CAD build for the part. Positions are in the model's coordinates, mm. A direction names the side the tool comes from. Round coordinates to 2 decimals unless told otherwise and drop trailing zeros. Order: outer loops, then holes, each group sorted by start corner. A loop starts at its lowest first (then second) coordinate and runs counter-clockwise, first axis right, second up.
```python
from build123d import *

# Parameters (mm, degrees)
SKETCH1_W           = 9.5
SKETCH1_H           = 16.65
BOSS_EXTRUDE1_DEPTH = 0.2
SKETCH1_3_W         = 0.5
SKETCH1_3_H         = 0.5
BOSS_EXTRUDE2_DEPTH = 2
SKETCH1_4_W         = 9.5
SKETCH1_4_H         = 14.9
SKETCH1_4_W_2       = 9.1
SKETCH1_4_H_2       = 14.5
BOSS_EXTRUDE3_DEPTH = 0.25
BOSS_EXTRUDE4_DEPTH = 2
SKETCH1_6_W         = 0.670753581
SKETCH1_6_H         = 1.75
SKETCH1_6_W_2       = 1.029246419
SKETCH1_6_H_2       = 0.5
SKETCH1_6_W_3       = 3.329246419
BOSS_EXTRUDE5_DEPTH = 2
FILLET1_R           = 0.1
BOSS_EXTRUDE6_DEPTH = 0.2
SKETCH1_10_W        = 3.329246419
SKETCH1_10_H        = 0.5
SKETCH1_10_W_2      = 0.670753581
SKETCH1_10_H_2      = 1.75
BOSS_EXTRUDE7_DEPTH = 2
CUT_EXTRUDE1_DEPTH  = 18.429429136


with BuildPart() as part:
    # Sketch1 → Boss-Extrude1 (new body)
    with BuildSketch(Plane(origin=(0, 0, 0), x_dir=(1, 0, 0), z_dir=(0, 1, 0))):
        with Locations((0, -0.875)):
            Rectangle(SKETCH1_W, SKETCH1_H)
        Polygon((-3.55, 6.25), (3.05, 6.25), (3.05, 5.75), (3.55, 5.75), (3.55, -5.75), (3.05, -5.75), (3.05, -6.25), (-3.05, -6.25), (-3.05, -5.75), (-3.55, -5.75), align=None, mode=Mode.SUBTRACT)
    extrude(amount=-BOSS_EXTRUDE1_DEPTH)

    # Sketch1_3 → Boss-Extrude2 (add)
    with BuildSketch(Plane(origin=(0, 0, 0), x_dir=(1, 0, 0), z_dir=(0, 1, 0))):
        with Locations((3.3, -6)):
            Rectangle(SKETCH1_3_W, SKETCH1_3_H)
        with Locations((3.3, 6)):
            Rectangle(SKETCH1_3_W, SKETCH1_3_H)
        with Locations((-3.3, -6)):
            Rectangle(SKETCH1_3_W, SKETCH1_3_H)
    extrude(amount=-BOSS_EXTRUDE2_DEPTH)

    # Sketch1_4 → Boss-Extrude3 (add)
    with BuildSketch(Plane(origin=(0, 0, 0), x_dir=(1, 0, 0), z_dir=(0, 1, 0))):
        Rectangle(SKETCH1_4_W, SKETCH1_4_H)
        Rectangle(SKETCH1_4_W_2, SKETCH1_4_H_2, mode=Mode.SUBTRACT)
    extrude(amount=BOSS_EXTRUDE3_DEPTH)

    # Sketch1_5 → Boss-Extrude4 (add)
    with BuildSketch(Plane(origin=(0, 0, 0), x_dir=(1, 0, 0), z_dir=(0, 1, 0))):
        Polygon((-4.75, 7.45), (-4.75, -7.45), (-3.05, -7.45), (-3.05, -6.25), (-3.55, -6.25), (-3.55, 6.25), (-3.05, 6.25), (-3.05, 7.45), align=None)
        Polygon((3.55, -6.25), (3.05, -6.25), (3.05, -6.95), (4.079246419, -6.95), (4.079246419, -7.45), (4.75, -7.45), (4.75, 7.45), (4.079246419, 7.45), (4.079246419, 6.95), (3.05, 6.95), (3.05, 6.25), (3.55, 6.25), align=None)
    extrude(amount=-BOSS_EXTRUDE4_DEPTH)

    # Sketch1_6 → Boss-Extrude5 (add)
    with BuildSketch(Plane(origin=(0, 0, 0), x_dir=(1, 0, 0), z_dir=(0, 1, 0))):
        with Locations((-4.41462321, -8.325)):
            Rectangle(SKETCH1_6_W, SKETCH1_6_H)
        with Locations((3.56462321, 7.2)):
            Rectangle(SKETCH1_6_W_2, SKETCH1_6_H_2)
        with Locations((2.41462321, -7.2)):
            Rectangle(SKETCH1_6_W_3, SKETCH1_6_H_2)
        with Locations((4.41462321, -8.325)):
            Rectangle(SKETCH1_6_W, SKETCH1_6_H)
    extrude(amount=-BOSS_EXTRUDE5_DEPTH)

    # Fillet1
    fillet1_edges = [part.edges().sort_by_distance(p)[0] for p in [
        (3.05, -1.1, 6.95),
    ]]
    fillet(fillet1_edges, radius=FILLET1_R)

    # Sketch1_9 → Boss-Extrude6 (add)
    with BuildSketch(Plane(origin=(0, 0, 0), x_dir=(1, 0, 0), z_dir=(0, 1, 0))):
        Polygon((-4.079246419, 9.2), (-4.079246419, 7.45), (-3.05, 7.45), (0, 7.45), (0.75, 7.45), (3.05, 7.45), (4.079246419, 7.45), (4.079246419, 8.7), (0.75, 8.7), (0.75, 9.2), align=None)
    extrude(amount=-BOSS_EXTRUDE6_DEPTH)

    # Sketch1_10 → Boss-Extrude7 (add)
    with BuildSketch(Plane(origin=(0, 0, 0), x_dir=(1, 0, 0), z_dir=(0, 1, 0))):
        with Locations((2.41462321, 8.95)):
            Rectangle(SKETCH1_10_W, SKETCH1_10_H)
        Polygon((4.75, 9.2), (4.079246419, 9.2), (4.079246419, 8.7), (4.079246419, 7.45), (4.75, 7.45), align=None)
        with Locations((-4.41462321, 8.325)):
            Rectangle(SKETCH1_10_W_2, SKETCH1_10_H_2)
    extrude(amount=-BOSS_EXTRUDE7_DEPTH)

    # Sketch6 → Cut-Extrude1 (cut, through all)
    with BuildSketch(Plane.XY.offset(7.45)):
        with BuildLine():
            Line((-4.079246419, -2), (-3.779246419, -2))
            Line((-3.779246419, -2), (-3.779246419, -1.8))
            ThreePointArc((-3.779246419, -1.8), (-3.808535741, -1.729289322), (-3.879246419, -1.7))
            Line((-3.879246419, -1.7), (-3.979246419, -1.7))
            ThreePointArc((-3.979246419, -1.7), (-4.049957097, -1.729289322), (-4.079246419, -1.8))
            Line((-4.079246419, -1.8), (-4.079246419, -2))
        make_face()
    cut_extrude1 = extrude(amount=-CUT_EXTRUDE1_DEPTH, mode=Mode.SUBTRACT)

    # Mirror1: Cut-Extrude1 across plane
    add(cut_extrude1.mirror(Plane(origin=(0, 0, 0), x_dir=(0, 0, 1), z_dir=(1, 0, 0))), mode=Mode.SUBTRACT)


solid = part.part
```
1. Cut at D-D, the plane x = -2.5. Write the cut outline in (y, z).
2. Drill centre lines: line 1 (X direction, y = -0.2, z = 6); line 2 (Z direction, x = 2.5, y = -1.5); line 3 (X direction, y = -1.75, z = 0.5). Where is each one in solid material? Low to high.
3. Mould opens along X. For faces 1 (the face through (-4, 0, 0)), 2 (the face through (0, 0, 8)), 3 (the face through (2, -1, -8.7)), 4 (the face through (4.75, -1, 0)) say: released by +X, released by -X, zero draft, split by the parting line, or undercut.
4. Cut at C-C, the plane x = 1.25. Write the cut outline in (y, z), and give its area (3 significant figures).
5. Cut at A-A, the plane z = -1.5. Write the cut outline in (x, y), and give its area (3 significant figures).
6. Pin check, flat tips, straight feed: P1, Ø0.8, axis at x = -3.5, y = -0.5, coming from the +Z side; P2, Ø0.9, axis at x = -2, z = 8.5, coming from the +Y side. Stop position of each tip, or through.
7. Tool access for faces 5 (the face through (3.6, -1.1, -7.45)), 6 (the face through (-3.55, -1, 0)), 7 (the face through (-3.05, -1, -7)), 8 (the face through (2, -1, 7.45)): list every direction of +Z, -Z, +X, -X, +Y, -Y with a clear straight run to the whole face (end or side of a thin tool).
Outcome:
1. outline: (-0.2, -9.2) - (0, -9.2) - (0, -7.45) - (0.25, -7.45) - (0.25, -7.25) - (0, -7.25) - (0, -6.25) - (-0.2, -6.25) - close; (-0.2, 6.25) - (0, 6.25) - (0, 7.25) - (0.25, 7.25) - (0.25, 7.45) - (0, 7.45) - (0, 9.2) - (-0.2, 9.2) - close
2. line 1: x = -4.75 to -3.05, 3.05 to 4.75
2. line 2: z = -9.2 to -8.7, 6.95 to 7.45
2. line 3: x = -4.75 to -4.07, -3.79 to -3.55, 3.55 to 3.79, 4.07 to 4.75
3. face 1: undercut
3. face 2: zero draft
3. face 3: undercut
3. face 4: released by +X
4. outline: (-2, -9.2) - (0, -9.2) - (0, -7.45) - (0.25, -7.45) - (0.25, -7.25) - (0, -7.25) - (0, -6.25) - (-0.2, -6.25) - (-0.2, -8.7) - (-2, -8.7) - close; (-2, 6.95) - (-0.2, 6.95) - (-0.2, 6.25) - (0, 6.25) - (0, 7.25) - (0.25, 7.25) - (0.25, 7.45) - (0, 7.45) - (0, 9.2) - (-0.2, 9.2) - (-0.2, 7.45) - (-2, 7.45) - close
4. area: 3.08 mm2
5. outline: (-4.75, -2) - (-4.08, -2) - (-4.08, -1.8) arc R0.1 cw to (-3.98, -1.7) - (-3.88, -1.7) arc R0.1 cw to (-3.78, -1.8) - (-3.78, -2) - (-3.55, -2) - (-3.55, 0) - (-4.55, 0) - (-4.55, 0.25) - (-4.75, 0.25) - close; (3.55, -2) - (3.78, -2) - (3.78, -1.8) arc R0.1 cw to (3.88, -1.7) - (3.98, -1.7) arc R0.1 cw to (4.08, -1.8) - (4.08, -2) - (4.75, -2) - (4.75, 0.25) - (4.55, 0.25) - (4.55, 0) - (3.55, 0) - close
5. area: 4.73 mm2
6. P1: stops at z = 9.2
6. P2: stops at y = 0
7. face 5: -Y
7. face 6: +Y, -Y
7. face 7: +Z, -Z, -Y
7. face 8: +Z, -Y
